Build history of the part. All positions in model axes, mm. A direction names the side the tool comes from. Coordinates: 2 decimals unless noted, no trailing zeros. Write each loop counter-clockwise with the first axis right and the second up, starting at its lowest first coordinate (ties: lowest second). Pieces come first, ordered by that corner, then holes.
from build123d import *

# Parameters (mm, degrees)
F0_W      = 200
F0_H      = 200
F1_DEPTH  = 180
F2_W      = 190
F2_H      = 190
F3_DEPTH  = 170
F4_W      = 50
F4_H      = 50
F5_DEPTH  = 8
F6_W      = 80
F6_H      = 30
F7_DEPTH  = 30
F8_W      = 74
F8_H      = 24
F9_DEPTH  = 25
F10_W     = 91
F10_H     = 91
F11_DEPTH = 25
F12_R     = 7.5
F13_DEPTH = 25


with BuildPart() as f1:
    # F0 (on Top) → F1 (new body)
    with BuildSketch(Plane.XY):
        Rectangle(F0_W, F0_H)
    extrude(amount=F1_DEPTH)

    # F2 (on face) → F3 (cut)
    with BuildSketch(Plane.XY.offset(180)):
        Rectangle(F2_W, F2_H)
    extrude(amount=-F3_DEPTH, mode=Mode.SUBTRACT)

    # F4 (on face) → F5 (cut)
    with BuildSketch(Plane.YZ.offset(100)):
        with Locations((0, 75)):
            Rectangle(F4_W, F4_H)
    extrude(amount=-F5_DEPTH, mode=Mode.SUBTRACT)

    # F6 (on face) → F7 (join)
    with BuildSketch(Plane.XY.offset(10)):
        with Locations((40, -63.405036)):
            Rectangle(F6_W, F6_H)
    extrude(amount=F7_DEPTH)

    # F8 (on face) → F9 (cut)
    with BuildSketch(Plane.XY.offset(40)):
        with Locations((40, -63.405036)):
            Rectangle(F8_W, F8_H)
    extrude(amount=-F9_DEPTH, mode=Mode.SUBTRACT)

    # F10 (on Top) → F11 (cut)
    with BuildSketch(Plane.XY):
        with Locations((-35.5, 4.5)):
            Rectangle(F10_W, F10_H)
    extrude(amount=F11_DEPTH, mode=Mode.SUBTRACT)

    # F12 (on face) → F13 (cut)
    with BuildSketch(Plane.YZ.offset(-95)):
        with Locations((0, 39.5)):
            Circle(F12_R)
    extrude(amount=-F13_DEPTH, mode=Mode.SUBTRACT)


solid = f1.part
(1) Slice it at D-D, the plane y = -29. List the corners of the cut face in (x, z), and give its area (3 significant figures).
(2) Flat gauge pins, fed straight in: P1, Ø1.5, axis at x = -72, y = -57.5, coming from the +Z side; P2, Ø7, axis at x = 54.5, y = -67, coming from the +Z side. Where does each tip first touch, or does it go through?
(3) 3-axis set-ups, long thin cutter, end or side, ignore diameter. For faces 1 (the flat face through (95, -1, 115)), 2 (the flat face through (-36, 50, 5)), 3 (the flat face through (21, 1, 0)): which of +Z, -Z, +X, -X, +Y, -Y reach the whole face in a straight line?
(4) Two-plate mould, pull along Z, no slides. Class faces 4 (the flat face through (-81, 4, 5)), 5 (the cylindrical face through (-97.46, -1.63, 32.18)), 6 (the flat face through (-8, -96, 180)): pulls with the +Z half, pulls with the -Z half, needs draft (parallel to the pull), parting line crosses it, or undercut.
(5) Slice it at C-C, the plane x = -43. List the corners of the cut face in (y, z).
(6) Probe L1, parallel to Y at x = 61, z = 39; L2, parallel to X at y = -77.5, z = 73. List the from-to ranges inside material, lowest first.
(7) Slice it at B-B, the plane y = 0. List the corners of the cut face in (x, z), and give its area (4 significant figures).
(8) Slice it at A-A, the plane z = 24. List the corners of the cut face in (x, y).
Results:
1. outline: (-100, 0) - (-81, 0) - (-81, 10) - (-95, 10) - (-95, 180) - (-100, 180) - close; (10, 0) - (100, 0) - (100, 180) - (95, 180) - (95, 10) - (10, 10) - close
1. area: 2,790 mm2
2. P1: stops at z = 10
2. P2: stops at z = 15
3. face 1: +Z
3. face 2: +Z, -Z
3. face 3: -Z, +X, -X, +Y, -Y
4. face 4: needs draft
4. face 5: undercut
4. face 6: pulls with the +Z half
5. outline: (-100, 0) - (-41, 0) - (-41, 10) - (-95, 10) - (-95, 180) - (-100, 180) - close; (50, 0) - (100, 0) - (100, 180) - (95, 180) - (95, 10) - (50, 10) - close
6. L1: y = -100 to -95, -78.41 to -75.41, -51.41 to -48.41, 95 to 100
6. L2: x = -100 to -95, 95 to 100
7. outline: (-100, 0) - (-81, 0) - (-81, 10) - (-95, 10) - (-95, 32) - (-100, 32) - close; (-100, 47) - (-95, 47) - (-95, 180) - (-100, 180) - close; (10, 0) - (100, 0) - (100, 50) - (95, 50) - (95, 10) - (10, 10) - close; (95, 100) - (100, 100) - (100, 180) - (95, 180) - close
7. area: 2,465 mm2
8. outline: (-100, -100) - (100, -100) - (100, 100) - (-100, 100) - close; (0, -78.41) - (80, -78.41) - (80, -48.41) - (0, -48.41) - close; hole (-95, -95) - (95, -95) - (95, 95) - (-95, 95) - close; hole (3, -75.41) - (77, -75.41) - (77, -51.41) - (3, -51.41) - close
